For this review, use the dimensioned drawing (mm, ordinates from the lowest corner) and the shaded views. Give positions to 0.01 mm unless a question says otherwise; leave off trailing zeros. Write each loop counter-clockwise with the first axis right and the second up, starting at its lowest first coordinate (ties: lowest second). Pieces come first, ordered by that corner, then holes.
1) We need section A-A on y = 5.1. Give the boundary of the cut face in (x, z), and give its area (3 significant figures).
2) We need section B-B on y = 4.05. Give the boundary of the cut face in (x, z), and give its area (3 significant figures).
3) Draft analysis for pull direction Z (two halves, no side actions). For the marked faces 1, 2 and 3, state which applies: pulls with the +Z half, pulls with the -Z half, needs draft (parallel to the pull), parting line crosses it, or undercut.
4) For P1, Ø1, axis at y = 2.5, z = 3.5, coming from the +X side; P2, Ø0.8, axis at x = 6, y = 5.5, coming from the -Z side, all flat-tipped, find the tip position at first contact; note any pin that passes through.
5) Wall thickness on line 1 along Z through (x, y) = (4.75, 1.1); line 2 along Z through (x, y) = (8.25, 4.75): over which ranges is each line inside the solid? List them lowest first.
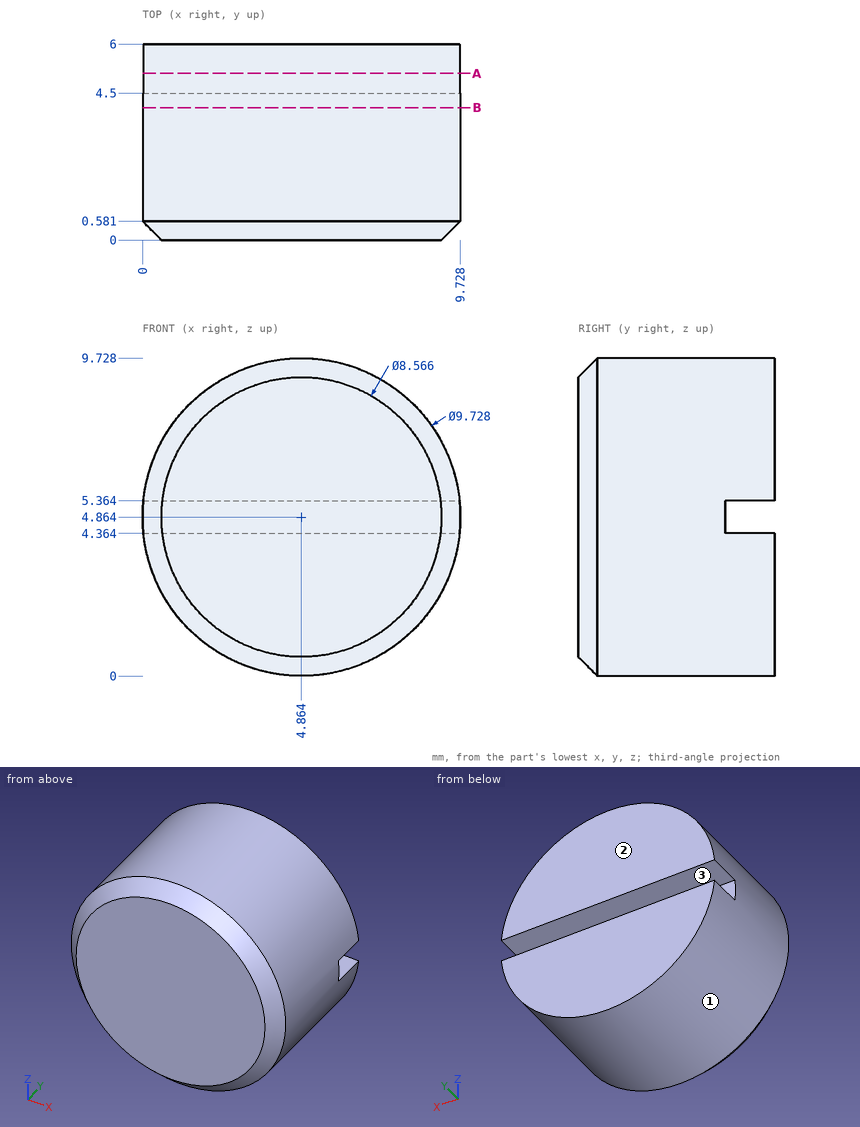
Results list:
1. outline: (0.03, 4.36) arc R4.86 ccw to (9.7, 4.36) - close; (0.03, 5.36) - (9.7, 5.36) arc R4.86 ccw to start
1. area: 64.6 mm2
2. outline: circle Ø9.73 at (4.86, 4.86)
2. area: 74.3 mm2
3. face 1: parting line crosses it
3. face 2: needs draft
3. face 3: undercut
4. P1: stops at x = 9.65
4. P2: stops at z = 0.06
5. line 1: z = 0 to 9.73
5. line 2: z = 1.37 to 4.36, 5.36 to 8.36
